```python
from build123d import *

# Parameters (mm, degrees)
F1_DEPTH = 12.7
F2_SIZE  = 6.34999
F4_D     = 22


# Not quite as in the source:
# - a fillet or chamfer is up to 0.001 mm smaller than in the source, because OpenCascade refuses the exact size


with BuildPart() as f1:
    # F0 (on Right) → F1 (new body)
    with BuildSketch(Plane.YZ):
        Polygon((0, 27.1703749895), (-51.3384975493, 46.6850064695), (-27.3204874247, 0), (0, 0), align=None)
        Polygon((0, 0), (-27.3204874247, 0), (-51.3384975493, -52.9897361994), (0, -26.5776470263), align=None)
        Polygon((23.7766716471, 0), (0, 0), (0, -26.5776470263), (51.0382726789, -52.9897361994), align=None)
        Polygon((51.0382726789, 46.6850064695), (0, 27.1703749895), (0, 0), (23.7766716471, 0), align=None)
    extrude(amount=F1_DEPTH)

    # F2 (size 6.35 in the source; OpenCascade refuses exactly that, so slightly less here)
    f2_edges = [f1.edges().sort_by_distance(p)[0] for p in [
        (12.7, -39.329492, 23.342503),
        (0, -39.329492, 23.342503),
        (0, -25.669249, 36.927691),
        (12.7, -25.669249, 36.927691),
        (0, -39.329492, -26.494868),
        (0, -25.669249, -39.783692),
        (12.7, -25.669249, -39.783692),
        (12.7, -39.329492, -26.494868),
        (0, 25.519136, -39.783692),
        (12.7, 25.519136, -39.783692),
        (0, 37.407472, -26.494868),
        (12.7, 37.407472, -26.494868),
        (0, 37.407472, 23.342503),
        (12.7, 37.407472, 23.342503),
        (0, 25.519136, 36.927691),
        (12.7, 25.519136, 36.927691),
    ]]
    chamfer(f2_edges, length=F2_SIZE)

    # F4 (through all)
    with Locations(Plane(origin=(0, 0, 0), x_dir=(0, 1, 0), z_dir=(-1, 0, 0))):
        with Locations((0, 0)):
            Hole(F4_D / 2)


solid = f1.part
```
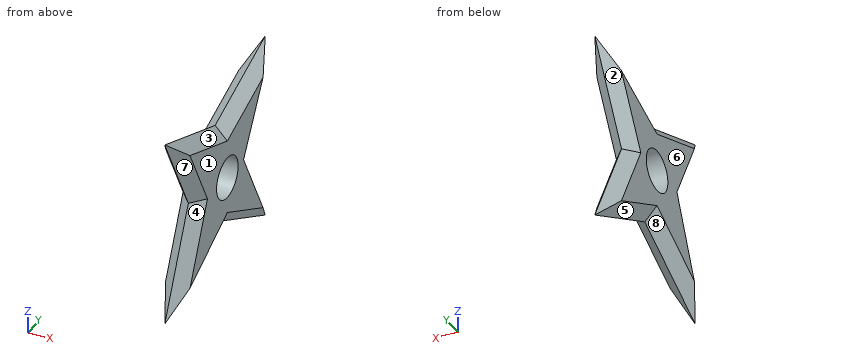
Input: part model. Units: mm. Frame: model coordinates. Face numbers are marked on the shaded views. A direction names the side the tool comes from. Round coordinates to 2 decimals unless told otherwise and drop trailing zeros. Loops run counter-clockwise (first coordinate to the right, second up) from the corner with the lowest first, then second, coordinate; pieces in that order, holes last. Notation, with made-up numbers: M 53.5,77 L 89.5,77 A26 cw 89.5,105 Z; hole C -32.75,1 d7. An arc over 180 degrees is marked long. Answer in a Markdown table with one row per item. Add a question column.
1. Set-up query: the marked faces 1, 2, 3, 4 and 5. Return all of +Z, -Z, +X, -X, +Y, -Y with unobstructed straight access to the full face (end or side cutting, diameter ignored); none if empty.
2. Section B-B (x = 3.25). Output: boundary loops of the cut face in (y, z).
3. Contact query for flat-ended pins moving along their axis: pin 1 (6 mm diameter, centred on x = 9.5, z = 3.5, fed in from -Y); pin 2 (5 mm diameter, centred on x = 11, y = -10.5, fed in from +Z); pin 3 (6 mm diameter, centred on x = 7.5, y = 22, fed in from +Z); pin 4 (10 mm diameter, centred on y = 27, z = -18, fed in from -X). Output: stop coordinate, or through.
4. Mould query, pull axis Z, two halves, no side actions, for the marked faces 6, 7 and 8. Classes: released by +Z, released by -Z, zero draft, split by the parting line, or undercut.
5. Ray query, probe 1 along Z at (x, y) = (11.25, 29.5); probe 2 along Z at (x, y) = (4, 41); probe 3 along Y at (x, z) = (3, -23). Return the intervals inside material, ascending.
Values follow:
| question | item | result |
|---|---|---|
| 1 | face 1 | +Z, -Z, +X, +Y, -Y |
| 1 | face 2 | -X, +Y |
| 1 | face 3 | +Z, +X |
| 1 | face 4 | +X, -Y |
| 1 | face 5 | -Z, -X |
| 2 | outline | M -44.88,40.92 L -23.88,0.09 L -44.84,-46.16 L 0,-23.09 L 43.84,-45.77 L 20.24,0.09 L 43.92,40.64 L 0,23.85 Z; hole C 0,0 d22 |
| 3 | pin 1 | y = -29.29 |
| 3 | pin 2 | z = 29.03 |
| 3 | pin 3 | z = 36.64 |
| 3 | pin 4 | x = 0 |
| 4 | face 6 | zero draft |
| 4 | face 7 | undercut |
| 4 | face 8 | released by -Z |
| 5 | probe 1 | -36.33 to -21.84, 19.52 to 33.2 |
| 5 | probe 2 | -45.15 to -38.61, 34.15 to 40.33 |
| 5 | probe 3 | -34.07 to -0.37, 0.38 to 31.84 |
